from build123d import *

# Parameters (mm, degrees)
SKETCH_1_R                    = 85
EXTRUDE_1_DEPTH               = 50
M14X1_5_1_D                   = 12.5
M14X1_5_1_DEPTH               = 34.5
M14X1_5_1_TIP                 = 3.755378869
HOLE_WIZARD_M12_1_D           = 13
HOLE_WIZARD_M12_1_CBORE_D     = 22
HOLE_WIZARD_M12_1_CBORE_DEPTH = 15
PATTERN_CIRCULAR_1_COUNT      = 8
SKETCH_6_W                    = 44.766058572
SKETCH_6_H                    = 9.083836387
SKETCH_6_H_2                  = 8.147377862
CUT_EXTRUDE_1_DEPTH           = 131.192165663
SKETCH_7_R                    = 16
CUT_EXTRUDE_2_DEPTH           = 20
SKETCH_8_R                    = 9
CUT_EXTRUDE_3_DEPTH           = 175.530799574
CHAMFER_1_SIZE                = 2
CHAMFER_2_SIZE                = 0.5


with BuildPart() as part:
    # 草圖1 → 填料-伸長1 (new body)
    with BuildSketch(Plane(origin=(0, 0, 0), x_dir=(1, 0, 0), z_dir=(0, 1, 0))):
        with Locations(Location((0, 0, 0), (0, 0, 270))):
            Circle(SKETCH_1_R)
    extrude(amount=EXTRUDE_1_DEPTH)

    # M14x1.5 螺紋孔1
    with Locations(Plane.XZ):
        with Locations((43, -27), (43, 27), (-43, 27), (-43, -27)):
            Hole(M14X1_5_1_D / 2, depth=M14X1_5_1_DEPTH)
            with Locations((0, 0, -(M14X1_5_1_DEPTH + M14X1_5_1_TIP / 2))):  # 118° drill point
                Cone(0, M14X1_5_1_D / 2, M14X1_5_1_TIP, mode=Mode.SUBTRACT)

    # M12 六角頭螺栓的柱孔1 (through all)
    with Locations(Plane.XZ):
        with Locations((-64.671567276, 26.787840266)):
            hole_wizard_m12_1 = CounterBoreHole(HOLE_WIZARD_M12_1_D / 2, HOLE_WIZARD_M12_1_CBORE_D / 2, HOLE_WIZARD_M12_1_CBORE_DEPTH)

    # 環狀複製排列1: M12 六角頭螺栓的柱孔1 ×8 about axis
    pattern_circular_1_axis = Axis((0, 0, 0), (0, 1, 0))
    for i in range(1, PATTERN_CIRCULAR_1_COUNT):
        add(hole_wizard_m12_1.rotate(pattern_circular_1_axis, i * 360 / PATTERN_CIRCULAR_1_COUNT), mode=Mode.SUBTRACT)

    # 草圖6 → 除料-伸長1 (cut, through all)
    with BuildSketch(Plane(origin=(0, 50, 0), x_dir=(1, 0, 0), z_dir=(0, 1, 0))):
        with Locations((0, 86.541918194)):
            Rectangle(SKETCH_6_W, SKETCH_6_H)
        with Locations((0, -86.073688931)):
            Rectangle(SKETCH_6_W, SKETCH_6_H_2)
    extrude(amount=-CUT_EXTRUDE_1_DEPTH, mode=Mode.SUBTRACT)

    # 草圖7 → 除料-伸長2 (cut)
    with BuildSketch(Plane(origin=(0, 0, -82), x_dir=(-1, 0, 0), z_dir=(0, 0, -1))):
        with Locations((0, 30)):
            Circle(SKETCH_7_R)
    cut_extrude_2 = extrude(amount=-CUT_EXTRUDE_2_DEPTH, mode=Mode.SUBTRACT)

    # 鏡射1: 除料-伸長2 across plane
    add(cut_extrude_2.mirror(Plane.XY), mode=Mode.SUBTRACT)

    # 草圖8 → 除料-伸長3 (cut, through all)
    with BuildSketch(Plane.XY.offset(62)):
        with Locations((0, 30)):
            Circle(SKETCH_8_R)
    extrude(amount=-CUT_EXTRUDE_3_DEPTH, mode=Mode.SUBTRACT)

    # 導角1
    chamfer_1_edges = [part.edges().sort_by_distance(p)[0] for p in [
        (-85, 50, 0),
        (-85, 0, 0),
        (85, 50, 0),
        (85, 0, 0),
    ]]
    chamfer(chamfer_1_edges, length=CHAMFER_1_SIZE)

    # 導角2
    chamfer_2_edges = [part.edges().sort_by_distance(p)[0] for p in [
        (-36.75, 0, 27),
        (49.25, 0, 27),
        (49.25, 0, -27),
        (-26.787840266, 0, -75.671567276),
    ]]
    chamfer(chamfer_2_edges, length=CHAMFER_2_SIZE)


solid = part.part
The listing builds one solid part. Answer for the finished solid, in the listing's coordinates (mm). A direction names the side the tool comes from. Coordinates: 2 decimals unless noted, no trailing zeros. Loops run counter-clockwise (first coordinate to the right, second up) from the corner with the lowest first, then second, coordinate; pieces in that order, holes last. Notation, with made-up numbers: (72, 63) -> (90, 63) arc R19 cw to (90, 93) -> close; hole circle Ø8 at (78, 5.5). An arc over 180 degrees is marked (long way). Write item = value, one per line. Start each with the question number.
1) Given pin 1 Ø19 at (x, y) = (0, 30) entering from +Z; pin 2 Ø24 at (x, z) = (61.5, -31) entering from -Y; pin 3 Ø20 at (x, z) = (-26.79, 64.67) entering from -Y; pin 4 Ø2 at (y, z) = (43.5, 44) entering from -X, each flat-ended and moving along its own axis, determine where each tip first touches the part or whether it passes through.
2) A cutting plane is placed at B-B (x = 0). Give the vertices of the cut face in (y, z), then the cut area to 3 significant figures.
3) A cutting plane is placed at A-A (y = 30). Count the separate pieces of the cut face and the enclosed holes in it, then the cut area to 3 significant figures.
4) A tool of negligible diameter and unlimited length cuts with its end or side. For faces 4 (the face through (83.303, 0.319, 1.651)), 5 (the face through (58, 15, 27)), from which of +Z, -Z, +X, -X, +Y, -Y can it reach the whole face along a straight path? Write none if from no direction.
5) Straight lines are drawn through the part: line 1 (Y direction, x = 0, z = 68.25); line 2 (X direction, y = 3, z = 61.5); line 3 (X direction, y = 25, z = 30.5). For each, find the intervals that lie inside material, in ascending order. Write a range as from..to.
6) The mould has two halves that part along Z. Classify faces 1 (the face through (1, 50, -1)), 2 (the face through (36.067, 7.395, -58.765)), 3 (the face through (-84.986, 24.678, -1.552)): released by +Z, released by -Z, zero draft, split by the parting line, or undercut.
Responses:
q1.pin_1 = 62
q1.pin_2 = 0
q1.pin_3 = 15
q1.pin_4 = -73.32
q2.outline = (0, -82) -> (14, -82) -> (14, -62) -> (21, -62) -> (21, 62) -> (14, 62) -> (14, 82) -> (0, 82) -> close; (39, -62) -> (46, -62) -> (46, -82) -> (50, -82) -> (50, 82) -> (46, 82) -> (46, 62) -> (39, 62) -> close
q2.area = 4,690 mm²
q3.separate_pieces = 2
q3.enclosed_holes = 12
q3.area = 17,500 mm²
q4.face_4 = +X, -Y
q4.face_5 = -Y
q5.line_1 = 0..14, 46..50
q5.line_2 = -58.67..-37.32, -16.25..16.25, 37.32..58.67
q5.line_3 = -79.34..-70.01, -59.34..-48.18, -37.82..-7.48, 7.48..37.82, 48.18..59.34, 70.01..79.34
q6.face_1 = zero draft
q6.face_2 = undercut
q6.face_3 = split by the parting line
